```python
from build123d import *

# Parameters (mm, degrees)
SKETCH1_R              = 6
BOSS_EXTRUDE1_DEPTH    = 180
SKETCH2_R              = 6
SKETCH2_R_2            = 4
CUT_EXTRUDE1_DEPTH     = 10
FILLET1_R              = 2
FILLET1_OF_MIRROR1_R   = 2
MOVE_START             = -180.0000001
MOVE_FACE1_2_OUTLINE_W = 16
MOVE_FACE1_2_OUTLINE_H = 16
MOVE_FACE1_2_OUTLINE_R = 4
MOVE_FACE1_2_DEPTH     = 12.0000001


with BuildPart() as part:
    # Sketch1 → Boss-Extrude1 (new, symmetric)
    with BuildSketch(Plane.XY):
        with Locations(Location((0, 0, 0), (0, 0, 180))):
            Circle(SKETCH1_R)
    extrude(amount=BOSS_EXTRUDE1_DEPTH, both=True)

    # Sketch2 → Cut-Extrude1 (cut)
    with BuildSketch(Plane.XY.offset(180)):
        with Locations(Location((0, 0, 0), (0, 0, 180))):
            Circle(SKETCH2_R)
        Circle(SKETCH2_R_2, mode=Mode.SUBTRACT)
    cut_extrude1 = extrude(amount=-CUT_EXTRUDE1_DEPTH, mode=Mode.SUBTRACT)

    # Fillet1
    fillet1_edges = [part.edges().sort_by_distance(p)[0] for p in [
        (6, 0, 170),
    ]]
    fillet(fillet1_edges, radius=FILLET1_R - 0.0001)  # a hair under: the kernel refuses the full size

    # Mirror1: Cut-Extrude1 across plane
    add(cut_extrude1.mirror(Plane.XY), mode=Mode.SUBTRACT)

    # Fillet1 of Mirror1
    fillet1_of_mirror1_edges = [part.edges().sort_by_distance(p)[0] for p in [
        (6, 0, -170),
    ]]
    fillet(fillet1_of_mirror1_edges, radius=FILLET1_OF_MIRROR1_R - 0.0001)  # a hair under: the kernel refuses the full size

    # Move Face1: read off the stored shape, not the designer's step
    # Move Face1 outline → Move Face1 (revolve, cut)
    with BuildSketch(Plane.XZ):
        with BuildLine():
            Line((6, -168), (6, -166))
            ThreePointArc((6, -166), (5.414213562, -167.414213562), (4, -168))
            Line((4, -168), (6, -168))
        make_face()
    revolve(axis=Axis((0, 0, 0), (0, 0, 1)), mode=Mode.SUBTRACT)

    # Move Face1 2 outline → Move Face1 2 (cut)
    with BuildSketch(Plane.XY.offset(MOVE_START)):
        Rectangle(MOVE_FACE1_2_OUTLINE_W, MOVE_FACE1_2_OUTLINE_H)
        Circle(MOVE_FACE1_2_OUTLINE_R, mode=Mode.SUBTRACT)
    extrude(amount=MOVE_FACE1_2_DEPTH, mode=Mode.SUBTRACT)


solid = part.part
```
Work out the finished part from the listing and answer in its coordinate system (mm). A direction names the side the tool comes from. Coordinates: 2 decimals unless noted, no trailing zeros. Loops run counter-clockwise (first coordinate to the right, second up) from the corner with the lowest first, then second, coordinate; pieces in that order, holes last. Notation, with made-up numbers: M 15,25 L 59,25 A14 cw 59,43 Z; hole C 65,67 d8. An arc over 180 degrees is marked long. Use CSV: the item, a comma, the result in double quotes. Start each with the question number.
(1) For faces 1 (the face through (-0.867, -3.905, 175.07)), 2 (the face through (-5.723, -1.802, 3.338)), determine the directions among +Z, -Z, +X, -X, +Y, -Y from which every point of the face is accessible in a straight line to the end or side of a thin tool.
(2) Consider line 1 (Z direction, x = -1, y = -4.25); line 2 (Y direction, x = 0.25, z = -111.5); line 3 (X direction, y = -4.5, z = -34.5). Determine where each line is inside the solid, lowest interval first.
(3) Given pin 1 Ø6 at (x, y) = (-3, -4.5) entering from -Z; pin 2 Ø1 at (x, z) = (3.5, -110.5) entering from +Y; pin 3 Ø6 at (y, z) = (4.5, 113) entering from +X; pin 4 Ø4 at (y, z) = (-3.5, -34.5) entering from -X, each flat-ended and moving along its own axis, determine where each tip first touches the part or whether it passes through.
(4) For a pull along Z with two mould halves and no side action, classify faces 3 (the face through (0, 0, -180)), 4 (the face through (0, 0, 180)), 5 (the face through (-0.867, -3.905, -174.084)) as +Z half, -Z half, draft (parallel to the pull), parting line (faces both ways), or undercut.
(5) Find section C-C, the plane z = 131. Give the vertices of the cut face in (x, y), then the cut area to 3 significant figures.
Recorded:
1,face 1,"+Z"
1,face 2,"+Z, -Z"
2,line 1,"z = -167.97 to 169.97"
2,line 2,"y = -5.99 to 5.99"
2,line 3,"x = -3.97 to 3.97"
3,pin 1,"stops at z = -180"
3,pin 2,"stops at y = 5.2"
3,pin 3,"stops at x = 5.81"
3,pin 4,"stops at x = -5.81"
4,face 3,"-Z half"
4,face 4,"+Z half"
4,face 5,"draft"
5,outline,"C 0,0 d12"
5,area,"113 mm^2"
